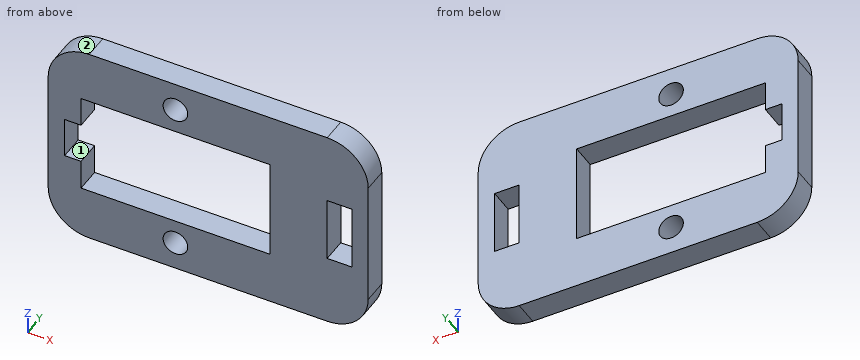
from build123d import *

# Parameters (mm, degrees)
ESBO_O1_R                = 1.5
RESSALTO_EXTRUS_O1_DEPTH = 3


with BuildPart() as part:
    # Esboço1 → Ressalto-extrusão1 (new body)
    with BuildSketch(Plane(origin=(0, 0, 0), x_dir=(1, 0, 0), z_dir=(0, 1, 0))):
        with BuildLine():
            Line((11.5, 6.5), (1, 6.5))
            ThreePointArc((1, 6.5), (-2.535533906, 5.035533906), (-4, 1.5))
            Line((-4, 1.5), (-4, -13.9))
            ThreePointArc((-4, -13.9), (-2.535533906, -17.435533906), (1, -18.9))
            Line((1, -18.9), (30, -18.9))
            ThreePointArc((30, -18.9), (33.535533906, -17.435533906), (35, -13.9))
            Line((35, -13.9), (35, 1.5))
            ThreePointArc((35, 1.5), (33.535533906, 5.035533906), (30, 6.5))
            Line((30, 6.5), (11.5, 6.5))
        make_face()
        with Locations(Location((11.5, 3, 0), (0, 0, 270))):
            Circle(ESBO_O1_R, mode=Mode.SUBTRACT)
        with Locations(Location((11.5, -15.4, 0), (0, 0, 90))):
            Circle(ESBO_O1_R, mode=Mode.SUBTRACT)
        Polygon((0, 0), (23, 0), (23, -12.4), (0, -12.4), (0, -8.7), (-2, -8.7), (-2, -3.7), (0, -3.7), align=None, mode=Mode.SUBTRACT)
        Polygon((30, -6.2), (30, -2.2), (33, -2.2), (33, -10.2), (30, -10.2), align=None, mode=Mode.SUBTRACT)
    extrude(amount=RESSALTO_EXTRUS_O1_DEPTH)


solid = part.part
For this review, take the finished solid that the model builds, in its own axes (mm). Face numbers are marked on the shaded views. A direction names the side the tool comes from. Coordinates: 2 decimals unless noted, no trailing zeros. Loops run counter-clockwise (first coordinate to the right, second up) from the corner with the lowest first, then second, coordinate; pieces in that order, holes last. Notation, with made-up numbers: (60.25, 15) - (94.25, 15) arc R28 ccw to (94.25, 48) - close; hole circle Ø5 at (28, 50.5). An arc over 180 degrees is marked (long way). Use a Markdown table: item, result. Add a question column.
Item 1: For line 1 (X direction, y = 0.35, z = 5); line 2 (X direction, y = 0.3, z = 3); line 3 (Z direction, x = 6, y = 2.6), list the stretches that pass through material, from the lowest coordinate up.
Item 2: We need section B-B (x = 11.5). Give the boundary of the cut face in (y, z).
Item 3: Insertion check: pin 1 Ø0.9 at (x, y) = (31, 2) entering from -Z; pin 2 Ø1.5 at (x, y) = (32, 2) entering from +Z. Each pin has a flat end and moves straight along its axis. Give the tip position at first contact, or say it passes through.
Item 4: Tool access review of the marked faces 1 and 2: name each direction out of +Z, -Z, +X, -X, +Y, -Y from which nothing blocks a thin tool from reaching the whole face with its end or side.
Item 5: We need section D-D (y = 1.55). Give the boundary of the cut face in (x, z).
Item 6: We need section A-A (x = 7). Give the boundary of the cut face in (y, z), and give its area (3 significant figures).
Item 7: We need section C-C (z = 1.25). Give the boundary of the cut face in (x, y).
Results list:
| question | item | result |
|---|---|---|
| 1 | line 1 | x = -4 to -2, 23 to 30, 33 to 35 |
| 1 | line 2 | x = -4 to 0, 23 to 30, 33 to 35 |
| 1 | line 3 | z = -6.5 to 0, 12.4 to 18.9 |
| 2 | outline | (0, -6.5) - (3, -6.5) - (3, -4.5) - (0, -4.5) - close; (0, -1.5) - (3, -1.5) - (3, 0) - (0, 0) - close; (0, 12.4) - (3, 12.4) - (3, 13.9) - (0, 13.9) - close; (0, 16.9) - (3, 16.9) - (3, 18.9) - (0, 18.9) - close |
| 3 | pin 1 | stops at z = -6.47 |
| 3 | pin 2 | stops at z = 18.74 |
| 4 | face 1 | +Y, -Y |
| 4 | face 2 | +Z, -X, +Y, -Y |
| 5 | outline | (-4, -1.5) arc R5 ccw to (1, -6.5) - (30, -6.5) arc R5 ccw to (35, -1.5) - (35, 13.9) arc R5 ccw to (30, 18.9) - (1, 18.9) arc R5 ccw to (-4, 13.9) - close; hole (-2, 3.7) - (0, 3.7) - (0, 0) - (23, 0) - (23, 12.4) - (0, 12.4) - (0, 8.7) - (-2, 8.7) - close; hole circle Ø3 at (11.5, -3); hole circle Ø3 at (11.5, 15.4); hole (30, 2.2) - (33, 2.2) - (33, 10.2) - (30, 10.2) - close |
| 6 | outline | (0, -6.5) - (3, -6.5) - (3, 0) - (0, 0) - close; (0, 12.4) - (3, 12.4) - (3, 18.9) - (0, 18.9) - close |
| 6 | area | 39.0 mm^2 |
| 7 | outline | (-4, 0) - (0, 0) - (0, 3) - (-4, 3) - close; (23, 0) - (35, 0) - (35, 3) - (23, 3) - close |
